Geometry: see drawing. Coordinates: mm, zero at the bounding-box minimum. Give positions to 0.01 mm unless a question says otherwise; leave off trailing zeros. Write each loop counter-clockwise with the first axis right and the second up, starting at its lowest first coordinate (ties: lowest second). Pieces come first, ordered by that corner, then holes. Notation, with made-up numbers: M 66,-10.5 L 79,-10.5 A20 ccw 79,0.5 Z; hole C 88.5,77 d6. An arc over 180 degrees is marked long. Use a Markdown table: item, result. Add a question column.
1) Section B-B on x = 10. Return the cut outline in (y, z), then the cut area to 3 significant figures.
2) Pin query (flat end, axial travel): pin 1 (6.5 mm diameter, centred on x = 10, z = 140, fed in from +Y). Return the tip coordinate at first contact, or that it passes through.
3) Line query: line 1 (X direction, y = 1.8, z = 140). Output: solid intervals per line, ascending.
4) Section A-A on z = 10. Return the cut outline in (x, y), then the cut area to 3 significant figures.
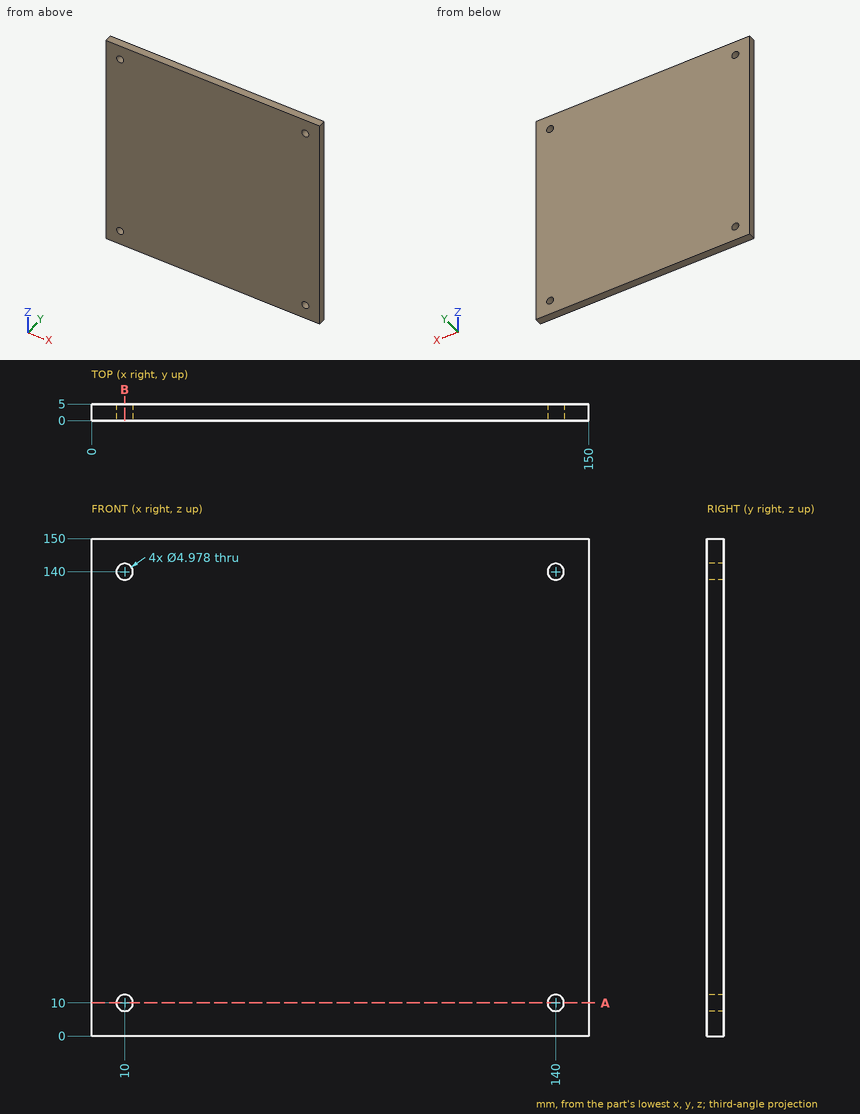
Found:
| question | item | result |
|---|---|---|
| 1 | outline | M 0,0 L 5,0 L 5,7.51 L 0,7.51 Z; M 0,12.49 L 5,12.49 L 5,137.51 L 0,137.51 Z; M 0,142.49 L 5,142.49 L 5,150 L 0,150 Z |
| 1 | area | 700 mm² |
| 2 | pin 1 | y = 5 |
| 3 | line 1 | 0 to 7.51, 12.49 to 137.51, 142.49 to 150 |
| 4 | outline | M 0,0 L 7.51,0 L 7.51,5 L 0,5 Z; M 12.49,0 L 137.51,0 L 137.51,5 L 12.49,5 Z; M 142.49,0 L 150,0 L 150,5 L 142.49,5 Z |
| 4 | area | 700 mm² |
